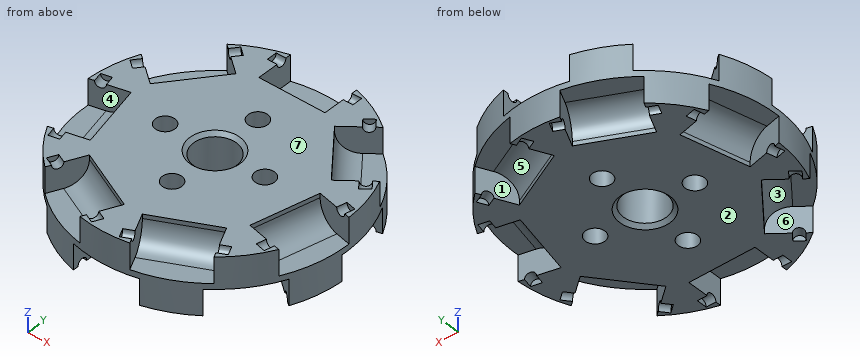
from build123d import *

# Parameters (mm, degrees)
SKETCH1_R           = 29.0703
BOSS_EXTRUDE2_DEPTH = 6.35
SKETCH2_W           = 14.732
SKETCH2_H           = 10.414
CUT_EXTRUDE2_DEPTH  = 5.715
CIRPATTERN1_COUNT   = 7
SKETCH4_R           = 1.143
CUT_EXTRUDE4_DEPTH  = 9.525
CIRPATTERN2_COUNT   = 7
SKETCH5_R           = 4.7625
CUT_EXTRUDE5_DEPTH  = 42.599124801
SKETCH6_R           = 2.159
CUT_EXTRUDE7_DEPTH  = 42.599124801
BOSS_EXTRUDE3_START = 6.35
SKETCH9_R           = 29.0703
SKETCH9_R_2         = 2.159
SKETCH9_R_3         = 4.7625
BOSS_EXTRUDE3_DEPTH = 6.35
CUT_EXTRUDE8_DEPTH  = 5.715
CIRPATTERN3_COUNT   = 7
SKETCH11_R          = 1.143
CUT_EXTRUDE9_DEPTH  = 9.525
CIRPATTERN4_COUNT   = 7
FILLET1_R           = 4.7625
CHAMFER1_SIZE       = 0.79375


with BuildPart() as part:
    # Sketch1 → Boss-Extrude2 (new body)
    with BuildSketch(Plane.XY):
        Circle(SKETCH1_R)
    extrude(amount=-BOSS_EXTRUDE2_DEPTH)

    # Sketch2 → Cut-Extrude2 (cut)
    with BuildSketch(Plane.XY):
        with Locations((0, 25.1333)):
            Rectangle(SKETCH2_W, SKETCH2_H)
    cut_extrude2 = extrude(amount=-CUT_EXTRUDE2_DEPTH, mode=Mode.SUBTRACT)

    # CirPattern1: Cut-Extrude2 ×7 about axis
    cirpattern1_axis = Axis((0, 0, 0), (0, 0, 1))
    for i in range(1, CIRPATTERN1_COUNT):
        add(cut_extrude2.rotate(cirpattern1_axis, i * 360 / CIRPATTERN1_COUNT), mode=Mode.SUBTRACT)

    # Sketch4 → Cut-Extrude4 (cut, symmetric)
    with BuildSketch(Plane(origin=(0, 0, 0), x_dir=(0, 0, -1), z_dir=(1, 0, 0))):
        with Locations((0, 25.7683)):
            Circle(SKETCH4_R)
    cut_extrude4 = extrude(amount=CUT_EXTRUDE4_DEPTH, both=True, mode=Mode.SUBTRACT)

    # CirPattern2: Cut-Extrude4 ×7 about axis
    cirpattern2_axis = Axis((0, 0, 0), (0, 0, 1))
    for i in range(1, CIRPATTERN2_COUNT):
        add(cut_extrude4.rotate(cirpattern2_axis, i * 360 / CIRPATTERN2_COUNT), mode=Mode.SUBTRACT)

    # Sketch5 → Cut-Extrude5 (cut, through all)
    with BuildSketch(Plane.XY):
        Circle(SKETCH5_R)
    extrude(amount=-CUT_EXTRUDE5_DEPTH, mode=Mode.SUBTRACT)

    # Sketch6 → Cut-Extrude7 (cut, through all)
    with BuildSketch(Plane(origin=(0, 0, -6.35), x_dir=(-1, 0, 0), z_dir=(0, 0, -1))):
        with Locations((0, 11.1125)):
            Circle(SKETCH6_R)
        with Locations((11.1125, 0)):
            Circle(SKETCH6_R)
        with Locations((0, -11.1125)):
            Circle(SKETCH6_R)
        with Locations((-11.1125, 0)):
            Circle(SKETCH6_R)
    extrude(amount=-CUT_EXTRUDE7_DEPTH, mode=Mode.SUBTRACT)

    # Sketch9 → Boss-Extrude3 (add)
    with BuildSketch(Plane(origin=(0, 0, -6.35), x_dir=(-1, 0, 0), z_dir=(0, 0, -1)).offset(BOSS_EXTRUDE3_START)):
        with Locations(Location((0, 0, 0), (0, 0, 178.179188094))):
            Circle(SKETCH9_R)
        with Locations((0, 11.1125)):
            Circle(SKETCH9_R_2, mode=Mode.SUBTRACT)
        with Locations((11.1125, 0)):
            Circle(SKETCH9_R_2, mode=Mode.SUBTRACT)
        with Locations((0, -11.1125)):
            Circle(SKETCH9_R_2, mode=Mode.SUBTRACT)
        with Locations((-11.1125, 0)):
            Circle(SKETCH9_R_2, mode=Mode.SUBTRACT)
        with Locations(Location((0, 0, 0), (0, 0, 180))):
            Circle(SKETCH9_R_3, mode=Mode.SUBTRACT)
    extrude(amount=-BOSS_EXTRUDE3_DEPTH)

    # Sketch10 → Cut-Extrude8 (cut)
    with BuildSketch(Plane(origin=(0, 0, -12.7), x_dir=(-1, 0, 0), z_dir=(0, 0, -1))):
        Polygon((-2.009055407, 21.148973594), (-15.282160644, 14.757064537), (-19.800579114, 24.139776859), (-6.527473878, 30.531685916), align=None)
    cut_extrude8 = extrude(amount=-CUT_EXTRUDE8_DEPTH, mode=Mode.SUBTRACT)

    # CirPattern3: Cut-Extrude8 ×7 about axis
    cirpattern3_axis = Axis((0, 0, 0), (0, 0, 1))
    for i in range(1, CIRPATTERN3_COUNT):
        add(cut_extrude8.rotate(cirpattern3_axis, i * 360 / CIRPATTERN3_COUNT), mode=Mode.SUBTRACT)

    # Sketch11 → Cut-Extrude9 (cut, symmetric)
    with BuildSketch(Plane(origin=(0, 0, 0), x_dir=(0, 0, -1), z_dir=(-0.900971031519736, 0.4338792462912495, 0))):
        with Locations((12.7, -25.7683)):
            Circle(SKETCH11_R)
    cut_extrude9 = extrude(amount=CUT_EXTRUDE9_DEPTH, both=True, mode=Mode.SUBTRACT)

    # CirPattern4: Cut-Extrude9 ×7 about axis
    cirpattern4_axis = Axis((0, 0, 0), (0, 0, 1))
    for i in range(1, CIRPATTERN4_COUNT):
        add(cut_extrude9.rotate(cirpattern4_axis, i * 360 / CIRPATTERN4_COUNT), mode=Mode.SUBTRACT)

    # Fillet1
    fillet1_edges = [part.edges().sort_by_distance(p)[0] for p in [
        (-15.579008669, 12.423844839, -5.715),
        (0, 19.9263, -5.715),
        (8.645608025, 17.953019065, -6.985),
        (-8.645787076, 17.952932839, -6.985),
        (-19.426728167, 4.433922012, -6.985),
        (-15.578946715, -12.423922526, -6.985),
        (9.9366e-05, -19.9263, -6.985),
        (15.579070622, -12.423767151, -6.985),
        (19.426683945, 4.434115761, -6.985),
        (8.645697551, -17.952975952, -5.715),
        (19.426706057, -4.434018886, -5.715),
        (-19.426706057, -4.434018886, -5.715),
        (-8.645697551, -17.952975952, -5.715),
        (15.579008669, 12.423844839, -5.715),
    ]]
    fillet(fillet1_edges, radius=FILLET1_R)

    # Chamfer1
    chamfer1_edges = [part.edges().sort_by_distance(p)[0] for p in [
        (-4.7625, 0, 0),
        (-4.7625, 0, -12.7),
    ]]
    chamfer(chamfer1_edges, length=CHAMFER1_SIZE)


solid = part.part
Design review of the part built by this model. Coordinates are the model's own, in mm. Face numbers are marked on the shaded views. A direction names the side the tool comes from. Coordinates: 2 decimals unless noted, no trailing zeros.
Item 1: Take a section at A-A, the plane z = -10. Count the separate pieces of the cut face and the enclosed holes in it, then the cut area to 3 significant figures.
Item 2: For pin 1 Ø7.5 at (x, y) = (9, -25) entering from +Z; pin 2 Ø1.5 at (x, y) = (22.5, -19.5) entering from -Z (3 decimals); pin 3 Ø4 at (y, z) = (15, -10.5) entering from +X, all flat-tipped, find the tip position at first contact; note any pin that passes through.
Item 3: For line 1 (Y direction, x = 0, z = -6); line 2 (X direction, y = 8, z = -4); line 3 (Y direction, x = 0, z = -4.25), list the stretches that pass through material, from the lowest coordinate up.
Item 4: For the marked faces 4, 5, 6 and 7, list the 3-axis set-ups (+Z, -Z, +X, -X, +Y, -Y) from which the entire face can be reached by the end or side of a thin tool; tool diameter is ignored.
Item 5: The part is to be moulded in two halves that separate along Y. For the marked faces 1, 2 and 3, say which applies: pulls with the +Y half, pulls with the -Y half, needs draft (parallel to the pull), parting line crosses it, or undercut.
The answers:
1. separate pieces: 1
1. enclosed holes: 5
1. area: 1,650 mm2
2. pin 1: stops at z = -5.27
2. pin 2: stops at z = -6.985
2. pin 3: stops at x = 25.78
3. line 1: y = -29.07 to -13.27, -8.95 to -4.76, 4.76 to 8.95, 13.27 to 29.07
3. line 2: x = -27.95 to -21.85, -20.52 to 20.52, 21.85 to 27.95
3. line 3: y = -29.07 to -13.27, -8.95 to -4.76, 4.76 to 8.95, 13.27 to 21.25
4. face 4: +Z
4. face 5: -Z
4. face 6: -Z, -X
4. face 7: +Z, +X, -X, +Y, -Y
5. face 1: pulls with the +Y half
5. face 2: needs draft
5. face 3: undercut
